```python
from build123d import *

# Parameters (mm, degrees)
ENL_V_MAT_EXTRU_3_DEPTH      = 285.465287865
R_P_TITION_CIRCULAIRE1_COUNT = 16
ENL_V_MAT_EXTRU_4_DEPTH      = 83.627706895


with BuildPart() as part:
    # Esquisse1 → R_volution1 (revolve)
    with BuildSketch(Plane.XY, mode=Mode.PRIVATE) as r_volution1_sk:
        Polygon((-198.5, 46), (-198.5, 0), (-150, 0), (0, 0), (0, 46), (-150, 46), align=None)
    revolve(r_volution1_sk.sketch.rotate(Axis((0, 46, 0), (0, -1, 0)), 270), axis=Axis((0, 46, 0), (0, -1, 0)))

    # Esquisse5 → Enl_v. mat.-Extru.3 (cut, through all)
    with BuildSketch(Plane(origin=(0, 46, 0), x_dir=(1, 0, 0), z_dir=(0, 1, 0))):
        Polygon((-37.5, 0), (-48.75, 0), (-198.5, 0), (-207.961569477, 0), (-202.600479892, 84.582990546), (-183.17739987, 76.474114423), (-44.986892915, 18.781426086), (-34.605302242, 14.447250836), (-36.059319151, 10.294440362), (-47.92540835, 8.928478843), (-48.53523435, 4.570943732), align=None)
    enl_v_mat_extru_3 = extrude(amount=-ENL_V_MAT_EXTRU_3_DEPTH, mode=Mode.SUBTRACT)

    # R_p_tition circulaire1: Enl_v. mat.-Extru.3 ×16 about axis
    r_p_tition_circulaire1_axis = Axis((0, 0, 0), (0, 1, 0))
    for i in range(1, R_P_TITION_CIRCULAIRE1_COUNT):
        add(enl_v_mat_extru_3.rotate(r_p_tition_circulaire1_axis, i * 360 / R_P_TITION_CIRCULAIRE1_COUNT), mode=Mode.SUBTRACT)

    # Esquisse6 → Enl_v. mat.-Extru.4 (cut, through all)
    with BuildSketch(Plane(origin=(0, 46, 0), x_dir=(1, 0, 0), z_dir=(0, 1, 0))):
        with BuildLine():
            Line((-12.296722124, 3.175), (-15.496722124, 3.175))
            Line((-15.496722124, 3.175), (-15.496722124, -3.175))
            Line((-15.496722124, -3.175), (-12.296722124, -3.175))
            ThreePointArc((-12.296722124, -3.175), (12.7, 0), (-12.296722124, 3.175))
        make_face()
    extrude(amount=-ENL_V_MAT_EXTRU_4_DEPTH, mode=Mode.SUBTRACT)


solid = part.part
```
Build history of the part. All positions in model axes, mm. A direction names the side the tool comes from. Coordinates: 2 decimals unless noted, no trailing zeros. Order: outer loops, then holes, each group sorted by start corner. A loop starts at its lowest first (then second) coordinate and runs counter-clockwise, first axis right, second up. Notation, with made-up numbers: M 21,39 L 43,39 A24 cw 43,52 Z; hole C 12,31.5 d4. An arc over 180 degrees is marked long. One line per question, with ' | ' between items. Start each with the question number.
1. Flat gauge pins, fed straight in: P1, Ø1.5, axis at y = 36.5, z = 15.5, coming from the -X side; P2, Ø9.5, axis at x = 42.5, y = 18, coming from the -Z side; P3, Ø4, axis at y = 19, z = 19.5, coming from the -X side; P4, Ø4, axis at x = -1.5, z = 13.5, coming from the -Y side. Where does each tip first touch, or does it go through?
2. Cut at B-B (z = -20.5). Write the cut outline in (x, y), plus the area to 3 significant figures.
3. Mould opens along X. For faces 1 (the face through (-6.78, 23.322, 48.226)), 2 (the face through (47.15, 23.32, -12.19)), 3 (the face through (14.351, 23, 41)) say: +X half, -X half, draft (parallel to the pull), parting line (faces both ways), or undercut.
4. Cut at A-A (x = 6.5). Write the cut outline in (y, z).
5. Tool access for faces 4 (the face through (38.9, 23.3, -29.3)), 5 (the face through (-37.38, 23.32, 2.06)), 6 (the face through (41.91, 23.32, 9.62)), 7 (the face through (-18.729, 23.322, 39.024)), 8 (the face through (-24.97, 23.32, 27.89)): list every direction of +Z, -Z, +X, -X, +Y, -Y with a clear straight run to the whole face (end or side of a thin tool).
6. Wall check: line 1 along Z through (x, y) = (0, 27); line 2 along X through (y, z) = (29, 0); line 3 along Z through (x, y) = (-41, 12.5). Give the ranges that are in metal, low to high. Write a range as [from, to].
7. Cut at C-C (x = -20.5). Write the cut outline in (y, z).
The answers:
1) P1: stops at x = -34.45 | P2: stops at z = -30.82 | P3: stops at x = -35.38 | P4: stops at y = 0
2) outline: M -40.79,0 L 34.59,0 L 34.59,46 L -40.79,46 Z | area: 3,470 mm2
3) face 1: -X half | face 2: +X half | face 3: undercut
4) outline: M 0,-48.27 L 46,-48.27 L 46,-10.91 L 0,-10.91 Z; M 0,10.91 L 46,10.91 L 46,41.23 L 0,41.23 Z
5) face 4: -Z, +X, +Y, -Y | face 5: -X, +Y, -Y | face 6: +X, +Y, -Y | face 7: +Z, +Y, -Y | face 8: +Y, -Y
6) line 1: z = [-37.49, -12.7], [12.7, 37.49] | line 2: x = [-37.49, -15.5], [12.7, 37.49] | line 3: z = [-26.35, -20.71], [-9.73, -1.45], [6.37, 14.35]
7) outline: M 0,-34.59 L 46,-34.59 L 46,40.79 L 0,40.79 Z
